from build123d import *

# Parameters (mm, degrees)
F1_DEPTH = 10.16
F3_DEPTH = 12.7
F5_D     = 3.429


with BuildPart() as f1:
    # F0 (on Front) → F1 (new body, symmetric)
    with BuildSketch(Plane.XZ):
        Polygon((0, 6.35), (-3.175, 6.35), (-6.35, 0), (0, 0), (6.35, 0), (3.175, 6.35), align=None)
    extrude(amount=F1_DEPTH, both=True)

    # F2 (on Right) → F3 (cut, symmetric)
    with BuildSketch(Plane.YZ):
        Polygon((-10.16, 6.35), (-10.16, 0), (-6.985, 6.35), align=None)
        Polygon((6.985, 6.35), (10.16, 0), (10.16, 6.35), align=None)
    extrude(amount=F3_DEPTH, both=True, mode=Mode.SUBTRACT)

    # F5 (through all)
    with Locations(Plane.XY.offset(6.35)):
        with Locations((0, 0)):
            Hole(F5_D / 2)


solid = f1.part
Design review of the part built by this model. Coordinates are the model's own, in mm. Round coordinates to 2 decimals unless told otherwise and drop trailing zeros. Write each loop counter-clockwise with the first axis right and the second up, starting at its lowest first coordinate (ties: lowest second). Pieces come first, ordered by that corner, then holes. Notation, with made-up numbers: (7, 13.25) - (13, 13.25) arc R26 cw to (13, 33.25) - close; hole circle Ø1 at (17, -39). An arc over 180 degrees is marked (long way). Return JSON: item names as keys, results as strings. Group by question number.
Item 1: For probe 1 along Y at (x, z) = (0, 4.5); probe 2 along Y at (x, z) = (0, 4.75) (1 decimal); probe 3 along X at (y, z) = (7.5, 1.25) (3 decimals), list the stretches that pass through material, from the lowest coordinate up. Write a range as [from, to].
Item 2: We need section D-D on z = 1.5. Write out the cut boundary in (x, y).
Item 3: The part is to be moulded in two halves that separate along Y. For faces 1 (the face through (0.372, -1.674, 3.131)), 2 (the face through (-1, -2, 6.35)), 3 (the face through (-0.09, -8.95, 2.42)), say which applies: pulls with the +Y half, pulls with the -Y half, needs draft (parallel to the pull), parting line crosses it, or undercut.
Item 4: We need section C-C on z = 3.5. Write out the cut boundary in (x, y).
Item 5: Insertion check: P1, Ø2.5, axis at x = 0, y = 0, coming from the -Z side; P2, Ø2, axis at x = 3.5, z = 2, coming from the +Y side. Each pin has a flat end and moves straight along its axis. Give the tip position at first contact, or say it passes through.
Model answer:
{
 "1": {"probe 1": "y = [-7.91, -1.71], [1.71, 7.91]", "probe 2": "y = [-7.8, -1.7], [1.7, 7.8]", "probe 3": "x = [-5.725, 5.725]"},
 "2": {"outline": "(-5.6, -9.41) - (5.6, -9.41) - (5.6, 9.41) - (-5.6, 9.41) - close; hole circle Ø3.43 at (0, 0)"},
 "3": {"face 1": "undercut", "face 2": "needs draft", "face 3": "pulls with the -Y half"},
 "4": {"outline": "(-4.6, -8.41) - (4.6, -8.41) - (4.6, 8.41) - (-4.6, 8.41) - close; hole circle Ø3.43 at (0, 0)"},
 "5": {"P1": "passes through", "P2": "stops at y = 9.66"}
}
